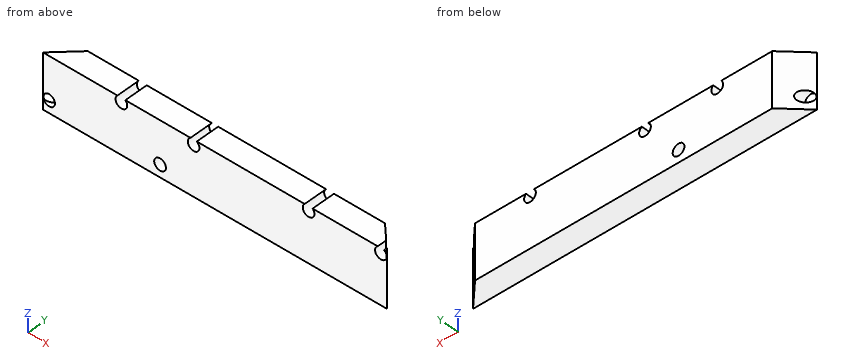
from build123d import *

# Parameters (mm, degrees)
SKETCH1_W                   = 560
SKETCH1_H                   = 88.9
BODY_DEPTH                  = 38.1
MOUNTING_HOLE_SPACING_REACH = 570.291
SKETCH2_R                   = 9.525
CUT_EXTRUDE1_REACH          = 570.291


with BuildPart() as part:
    # Sketch1 → Body (new body)
    with BuildSketch(Plane(origin=(0, 0, 0), x_dir=(1, 0, 0), z_dir=(0, 1, 0))):
        with Locations((280, 44.45)):
            Rectangle(SKETCH1_W, SKETCH1_H)
    extrude(amount=BODY_DEPTH)

    # Sketch2 → Mounting hole spacing (cut, up to next)
    with BuildSketch(Plane(origin=(0, 38.1, 0), x_dir=(1, 0, 0), z_dir=(0, 1, 0)), mode=Mode.PRIVATE) as mounting_hole_spacing_sk1:
        with Locations((127.6, 7)):
            Circle(SKETCH2_R)
    mounting_hole_spacing_tool1 = extrude(mounting_hole_spacing_sk1.sketch, amount=-MOUNTING_HOLE_SPACING_REACH, mode=Mode.PRIVATE) & part.part
    # Sketch2 → Mounting hole spacing (cut, up to next)
    with BuildSketch(Plane(origin=(0, 38.1, 0), x_dir=(1, 0, 0), z_dir=(0, 1, 0)), mode=Mode.PRIVATE) as mounting_hole_spacing_sk2:
        with Locations(Location((190.57, 68.87, 0), (0, 0, 270))):
            Circle(SKETCH2_R)
    mounting_hole_spacing_tool2 = extrude(mounting_hole_spacing_sk2.sketch, amount=-MOUNTING_HOLE_SPACING_REACH, mode=Mode.PRIVATE) & part.part
    # Sketch2 → Mounting hole spacing (cut, up to next)
    with BuildSketch(Plane(origin=(0, 38.1, 0), x_dir=(1, 0, 0), z_dir=(0, 1, 0)), mode=Mode.PRIVATE) as mounting_hole_spacing_sk3:
        with Locations(Location((10, 68.87, 0), (0, 0, 270))):
            Circle(SKETCH2_R)
    mounting_hole_spacing_tool3 = extrude(mounting_hole_spacing_sk3.sketch, amount=-MOUNTING_HOLE_SPACING_REACH, mode=Mode.PRIVATE) & part.part
    # Sketch2 → Mounting hole spacing (cut, up to next)
    with BuildSketch(Plane(origin=(0, 38.1, 0), x_dir=(1, 0, 0), z_dir=(0, 1, 0)), mode=Mode.PRIVATE) as mounting_hole_spacing_sk4:
        with Locations((245.2, 8.02)):
            Circle(SKETCH2_R)
    mounting_hole_spacing_tool4 = extrude(mounting_hole_spacing_sk4.sketch, amount=-MOUNTING_HOLE_SPACING_REACH, mode=Mode.PRIVATE) & part.part
    # Sketch2 → Mounting hole spacing (cut, up to next)
    with BuildSketch(Plane(origin=(0, 38.1, 0), x_dir=(1, 0, 0), z_dir=(0, 1, 0)), mode=Mode.PRIVATE) as mounting_hole_spacing_sk5:
        with Locations((550, 8.02)):
            Circle(SKETCH2_R)
    mounting_hole_spacing_tool5 = extrude(mounting_hole_spacing_sk5.sketch, amount=-MOUNTING_HOLE_SPACING_REACH, mode=Mode.PRIVATE) & part.part
    # Sketch2 → Mounting hole spacing (cut, up to next)
    with BuildSketch(Plane(origin=(0, 38.1, 0), x_dir=(1, 0, 0), z_dir=(0, 1, 0)), mode=Mode.PRIVATE) as mounting_hole_spacing_sk6:
        with Locations((432.4, 7)):
            Circle(SKETCH2_R)
    mounting_hole_spacing_tool6 = extrude(mounting_hole_spacing_sk6.sketch, amount=-MOUNTING_HOLE_SPACING_REACH, mode=Mode.PRIVATE) & part.part
    add(mounting_hole_spacing_tool1.solids().sort_by_distance((127.6, 38.1, -7))[0], mode=Mode.SUBTRACT)
    add(mounting_hole_spacing_tool2.solids().sort_by_distance((190.57, 38.1, -68.87))[0], mode=Mode.SUBTRACT)
    add(mounting_hole_spacing_tool3.solids().sort_by_distance((10, 38.1, -68.87))[0], mode=Mode.SUBTRACT)
    add(mounting_hole_spacing_tool4.solids().sort_by_distance((245.2, 38.1, -8.02))[0], mode=Mode.SUBTRACT)
    add(mounting_hole_spacing_tool5.solids().sort_by_distance((550, 38.1, -8.02))[0], mode=Mode.SUBTRACT)
    add(mounting_hole_spacing_tool6.solids().sort_by_distance((432.4, 38.1, -7))[0], mode=Mode.SUBTRACT)

    # Sketch3 → Cut-Extrude1 (cut, up to next)
    with BuildSketch(Plane(origin=(0, 0, -88.9), x_dir=(-1, 0, 0), z_dir=(0, 0, -1)), mode=Mode.PRIVATE) as cut_extrude1_sk1:
        Polygon((-560, 0), (-521.9, 38.1), (-560, 38.1), align=None)
    cut_extrude1_tool1 = extrude(cut_extrude1_sk1.sketch, amount=-CUT_EXTRUDE1_REACH, mode=Mode.PRIVATE) & part.part
    # Sketch3 → Cut-Extrude1 (cut, up to next)
    with BuildSketch(Plane(origin=(0, 0, -88.9), x_dir=(-1, 0, 0), z_dir=(0, 0, -1)), mode=Mode.PRIVATE) as cut_extrude1_sk2:
        Polygon((0, 38.1), (0, 0), (-38.1, 38.1), align=None)
    cut_extrude1_tool2 = extrude(cut_extrude1_sk2.sketch, amount=-CUT_EXTRUDE1_REACH, mode=Mode.PRIVATE) & part.part
    add(cut_extrude1_tool1.solids().sort_by_distance((547.3, 25.4, -88.9))[0], mode=Mode.SUBTRACT)
    add(cut_extrude1_tool2.solids().sort_by_distance((12.7, 25.4, -88.9))[0], mode=Mode.SUBTRACT)


solid = part.part
Design review of the part built by this model. Coordinates are the model's own, in mm. Round coordinates to 2 decimals unless told otherwise and drop trailing zeros. Order: outer loops, then holes, each group sorted by start corner. A loop starts at its lowest first (then second) coordinate and runs counter-clockwise, first axis right, second up.
1) Clearance check with flat-ended pins moving along their axes: pin 1 Ø12 at (y, z) = (10.5, -62) entering from -X; pin 2 Ø1 at (y, z) = (4.5, -71) entering from -X; pin 3 Ø8 at (y, z) = (9, -21.5) entering from -X; pin 4 Ø3 at (x, z) = (337.5, -16.5) entering from -Y. State where each tip first meets the part, or that it passes through.
The answers:
pin 1: stops at x = 4.58
pin 2: stops at x = 19.15
pin 3: stops at x = 5
pin 4: stops at y = 0
2) Consider section D-D (z = -11). State the section outline as (x, y) points, plus the area to 3 significant figures.
The answers:
outline: (0, 0) - (118.96, 0) - (118.96, 38.1) - (38.1, 38.1) - close; (136.24, 0) - (236.15, 0) - (236.15, 38.1) - (136.24, 38.1) - close; (254.25, 0) - (423.76, 0) - (423.76, 38.1) - (254.25, 38.1) - close; (441.04, 0) - (540.95, 0) - (540.95, 19.05) - (521.9, 38.1) - (441.04, 38.1) - close; (559.05, 0) - (560, 0) - (559.05, 0.95) - close
area: 17,700 mm2
3) For L1, parallel to X at y = 29, z = -7 (3 decimals); L2, parallel to Z at x = 190, y = 30; L3, parallel to X at y = 34.5, z = -9, list the stretches that pass through material, from the lowest coordinate up.
The answers:
L1: x = 29 to 118.075, 137.125 to 235.73, 254.67 to 422.875, 441.925 to 531
L2: z = -88.9 to -78.38, -59.36 to 0
L3: x = 34.5 to 118.29, 136.91 to 235.73, 254.67 to 423.09, 441.71 to 525.5
4) Consider section C-C (z = -68.87). State the section outline as (x, y) points (3 decimals), plus the area to 3 significant figures.
The answers:
outline: (0, 0) - (0.475, 0) - (0.475, 0.475) - close; (19.525, 0) - (181.045, 0) - (181.045, 38.1) - (38.1, 38.1) - (19.525, 19.525) - close; (200.095, 0) - (560, 0) - (521.9, 38.1) - (200.095, 38.1) - close
area: 19,000 mm2
5) Consider section A-A (y = 26.5). State the section outline as (x, z) points (3 decimals).
The answers:
outline: (26.5, -88.9) - (533.5, -88.9) - (533.5, 0) - (438.86, 0) arc R9.525 cw (long way) to (425.94, 0) - (250.339, 0) arc R9.525 cw (long way) to (240.061, 0) - (134.06, 0) arc R9.525 cw (long way) to (121.14, 0) - (26.5, 0) - close; hole circle Ø19.05 at (190.57, -68.87)
6) Consider section B-B (x = 10). State the section outline as (y, z) points (3 decimals), plus the area to 4 significant figures.
The answers:
outline: (0, -88.9) - (10, -88.9) - (10, -78.395) - (0, -78.395) - close; (0, -59.345) - (10, -59.345) - (10, 0) - (0, 0) - close
area: 698.5 mm2
